from build123d import *

# Parameters (mm, degrees)
ESQUISSE1_R                  = 10
BOSS_EXTRU_1_DEPTH           = 15
ESQUISSE2_R                  = 2.85
ESQUISSE2_R_2                = 2.35
ENL_V_MAT_EXTRU_1_DEPTH      = 1
ESQUISSE3_R                  = 1.25
ENL_V_MAT_EXTRU_2_DEPTH      = 16
ESQUISSE4_W                  = 5
ESQUISSE4_H                  = 5
ENL_V_MAT_EXTRU_3_DEPTH      = 11
ENL_V_MAT_EXTRU_3_DEPTH_BACK = 11


with BuildPart() as part:
    # Esquisse1 → Boss.-Extru.1 (new body)
    with BuildSketch(Plane(origin=(0, 0, 0), x_dir=(1, 0, 0), z_dir=(0, 1, 0))):
        Circle(ESQUISSE1_R)
    extrude(amount=BOSS_EXTRU_1_DEPTH)

    # Esquisse2 → Enlèv. mat.-Extru.1 (cut)
    with BuildSketch(Plane(origin=(0, 15, 0), x_dir=(1, 0, 0), z_dir=(0, 1, 0))):
        Circle(ESQUISSE2_R)
        Circle(ESQUISSE2_R_2, mode=Mode.SUBTRACT)
    extrude(amount=-ENL_V_MAT_EXTRU_1_DEPTH, mode=Mode.SUBTRACT)

    # Esquisse3 → Enlèv. mat.-Extru.2 (cut, through all)
    with BuildSketch(Plane(origin=(0, 15, 0), x_dir=(1, 0, 0), z_dir=(0, 1, 0))):
        Circle(ESQUISSE3_R)
    extrude(amount=-ENL_V_MAT_EXTRU_2_DEPTH, mode=Mode.SUBTRACT)

    # Esquisse4 → Enlèv. mat.-Extru.3 (cut, two sides)
    with BuildSketch(Plane(origin=(0, 0, 0), x_dir=(0, 0, -1), z_dir=(1, 0, 0))) as enl_v_mat_extru_3_sk:
        with Locations((-7.5, 7.5)):
            Rectangle(ESQUISSE4_W, ESQUISSE4_H)
        with Locations((7.5, 7.5)):
            Rectangle(ESQUISSE4_W, ESQUISSE4_H)
    extrude(amount=ENL_V_MAT_EXTRU_3_DEPTH, mode=Mode.SUBTRACT)
    extrude(enl_v_mat_extru_3_sk.sketch, amount=-ENL_V_MAT_EXTRU_3_DEPTH_BACK, mode=Mode.SUBTRACT)


solid = part.part
Could you check a few things on this model? Use its own coordinates, in mm. A direction names the side the tool comes from. Coordinates: 2 decimals unless noted, no trailing zeros. Write each loop counter-clockwise with the first axis right and the second up, starting at its lowest first coordinate (ties: lowest second). Pieces come first, ordered by that corner, then holes. Notation, with made-up numbers: (65, -19.75) - (122, -19.75) arc R27 ccw to (122, 12.25) - close; hole circle Ø6 at (23, 40). An arc over 180 degrees is marked (long way). Write item = value, one per line.
1) Please list where these lines run through material, in increasing order: line 1 (Z direction, x = 0, y = 7); line 2 (Z direction, x = 0, y = 14.75); line 3 (X direction, y = 9.25, z = 0). Write a range as [from, to].
Result set:
line_1 = [-5, -1.25], [1.25, 5]
line_2 = [-10, -2.85], [-2.35, -1.25], [1.25, 2.35], [2.85, 10]
line_3 = [-10, -1.25], [1.25, 10]
2) For faces 4 (the flat face through (0, 10, -7)), 5 (the cylindrical face through (-0.509, 14.507, 2.294)), 6 (the flat face through (0, 7, 5)), 7 (the flat face through (2, 0, 0)), which set-ups out of +Z, -Z, +X, -X, +Y, -Y let a thin tool reach every point of the face, with its end or its side?
Result set:
face_4 = -Z, +X, -X
face_5 = +Y
face_6 = +Z, +X, -X
face_7 = +Z, -Z, +X, -X, -Y
3) Suppose I cut it at C-C on y = 9. Please give me the cut outline in (x, z), plus the area to 3 significant figures.
Result set:
outline = (-8.66, -5) - (8.66, -5) arc R10 ccw to (8.66, 5) - (-8.66, 5) arc R10 ccw to start; hole circle Ø2.5 at (0, 0)
area = 186 mm2
4) Will these pins go through, and if not, where does the flat tip stop? pin 1 Ø5 at (y, z) = (11, -7) entering from -X; pin 2 Ø2.5 at (x, y) = (-4.5, 8.5) entering from -Z; pin 3 Ø5.5 at (x, y) = (3.5, 6.5) entering from +Z.
Result set:
pin_1 = -8.93
pin_2 = -5
pin_3 = 9.93
5) Suppose I cut it at B-B on x = 0. Please give me the cut outline in (y, z).
Result set:
outline = (0, -10) - (5, -10) - (5, -5) - (10, -5) - (10, -10) - (15, -10) - (15, -2.85) - (14, -2.85) - (14, -2.35) - (15, -2.35) - (15, -1.25) - (0, -1.25) - close; (0, 1.25) - (15, 1.25) - (15, 2.35) - (14, 2.35) - (14, 2.85) - (15, 2.85) - (15, 10) - (10, 10) - (10, 5) - (5, 5) - (5, 10) - (0, 10) - close
6) Suppose I cut it at A-A on z = 0. Please give me the cut outline in (x, y).
Result set:
outline = (-10, 0) - (-1.25, 0) - (-1.25, 15) - (-2.35, 15) - (-2.35, 14) - (-2.85, 14) - (-2.85, 15) - (-10, 15) - close; (1.25, 0) - (10, 0) - (10, 15) - (2.85, 15) - (2.85, 14) - (2.35, 14) - (2.35, 15) - (1.25, 15) - close
7) Suppose I cut it at D-D on x = 8.25. Please give me the cut outline in (y, z), plus the area to 3 significant figures.
Result set:
outline = (0, -5.65) - (5, -5.65) - (5, -5) - (10, -5) - (10, -5.65) - (15, -5.65) - (15, 5.65) - (10, 5.65) - (10, 5) - (5, 5) - (5, 5.65) - (0, 5.65) - close
area = 163 mm2
8) We'd pull the mould along Z, two halves only. Please class faces 1 (the flat face through (0, 7, -5)), 2 (the cylindrical face through (-0.27, 7.6, 1.22)), 3 (the cylindrical face through (9.237, 7.395, 3.83)): +Z half, -Z half, draft (parallel to the pull), parting line (faces both ways), or undercut.
Result set:
face_1 = -Z half
face_2 = undercut
face_3 = parting line
